Autodesk Inventor part; units mm, degrees
ref_plane "YZ Plane" through (0, 0, 0) normal (1, 0, 0) x (0, 1, 0)
ref_plane "XZ Plane" through (0, 0, 0) normal (0, 1, 0) x (-1, 0, 0)
ref_plane "XY Plane" through (0, 0, 0) normal (0, 0, 1) x (1, 0, 0)
sketch "Sketch1" plane through (0, 0, 0) normal (0, 0, 1) x (1, 0, 0)
  arc A0 (10, 32.7) -> (-10, 32.7) centre (0, 32.7) ccw
  line L0 (-10, 32.7) -> (-26, 14)
  line L1 (-26, 14) -> (-26, 7)
  line L2 (-26, 7) -> (-40, 7)
  line L3 (-40, 7) -> (-40, 0)
  line L4 (-40, 0) -> (0, 0)
  line L5 (0, 32.7) -> (0, 0) construction
  line L6 (10, 32.7) -> (26, 14)
  line L7 (26, 14) -> (26, 7)
  line L8 (26, 7) -> (40, 7)
  line L9 (40, 7) -> (40, 0)
  line L10 (40, 0) -> (0, 0)
  line L11 (-10, 32.7) -> (10, 32.7) construction
  dimension "d4" = 10
  dimension "d5" = 80
  dimension "ToolGuidance_Base_Thickness" = 7
  dimension "d7" = 7
  dimension "d8" = 32.7
  dimension "d9" = 14
  dimension "d11" = 0
extrude "Extrusion1" add sketch "Sketch1" against normal blind 60
sketch "Sketch2" plane through (0, 0, 0) normal (0, 0, 1) x (1, 0, 0)
  arc A0 (10, 32.7) -> (-10, 32.7) centre (0, 32.7) ccw
  circle A1 centre (0, 32.7) radius 8
  point P0 (0, 0)
  dimension "d16" = 16
extrude "Extrusion2" cut sketch "Sketch2" against normal blind 20
sketch "Sketch3" plane through (0, 0, -60) normal (0, 0, -1) x (-1, 0, 0)
  circle A0 centre (0, 32.7) radius 8
  circle A1 centre (0, 32.7) radius 4.25
  point P0 (0, 0)
  dimension "d19" = 8.5
extrude "Extrusion3" cut sketch "Sketch3" against normal blind 60 contours A1
sketch "Sketch4" plane through (-40, 7, 0) normal (0, 1, 0) x (1, 0, 0)
  circle A0 centre (5, 52) radius 2.25 construction
  line L0 (0, 60) -> (14, 60) construction
  line L1 (0, 0) -> (0, 60) construction
  circle A1 centre (5, 8) radius 2.25 construction
  line L2 (96, 0) -> (-16, 0) construction
  line L3 (40, 60) -> (40, 0) construction
  circle A2 centre (75, 52) radius 2.25 construction
  circle A3 centre (75, 8) radius 2.25 construction
  line L4 (80, 0) -> (80, 60) construction
  line L5 (66, 60) -> (80, 60) construction
  line L6 (75, 52) -> (75, 8) construction
  line L7 (5, 52) -> (5, 8) construction
  line L8 (0, 0) -> (0, 60) construction
  point P0 (73, 60)
  point P1 (7, 60)
  dimension "d25" = 4.5
  dimension "d26" = 8
  dimension "d28" = 4.5
  dimension "d29" = 8
  dimension "d54" = 44
  dimension "Guidacne_fixHoleDist" = 70
hole "Bohrung1" at (35, 7, -52) at (35, 7, -8) at (-35, 7, -8) at (-35, 7, -52) direction (0, -1, 0) diameter 3.4 end through all counterbore diameter 6.5 counterbore depth 3.4
sketch "Sketch5" plane through (0, 0, 0) normal (1, 0, 0) x (0, 1, 0)
  line L0 (32.7, 0) -> (32.7, -60)
  line L1 (32.7, 0) -> (32.7, -180.9299)
  line L2 (32.7, -60) -> (42.7, -60)
  line L3 (42.7, -60) -> (38.95, -110)
  line L4 (38.95, -110) -> (38.95, -155)
  line L5 (36.95, -60) -> (36.95, -20)
  line L6 (36.95, -60) -> (36.95, -155)
  line L7 (36.95, -155) -> (38.95, -155)
  line L8 (42.7, 0) -> (32.7, 0)
  point P0 (0, 0)
  dimension "d34" = 2
  dimension "d35" = 155
  dimension "d36" = 110
revolve "Revolution1" add sketch "Sketch5" angle 360 about axis through (0, 32.7, 0) along (0, 0, -1)
sketch "Sketch6" plane through (0, 0, 0) normal (1, 0, 0) x (0, 1, 0)
  line L0 (32.7, 0) -> (32.7, -60)
  line L1 (32.7, -41.8536) -> (32.7, 16.9969)
  line L2 (24.7, -20) -> (40.7, -20)
  line L3 (40.7, -20) -> (36.95, -33.9952)
  line L4 (36.95, -155) -> (36.95, -20)
  line L5 (28.45, -20) -> (36.95, -20)
  line L6 (36.95, -33.9952) -> (36.95, -20)
  line L7 (36.95, -20) -> (40.7, -20)
  line L8 (36.95, -33.9952) -> (36.95, -20)
  line L9 (40.7, -20) -> (36.95, -20)
  point P0 (0, 0)
  dimension "d38" = 15
revolve "Revolution2" cut sketch "Sketch6" angle 360 about axis through (0, 32.7, -41.8536) along (0, 0, 1)
sketch "Sketch7" plane through (0, 0, 0) normal (1, 0, 0) x (0, 1, 0)
  line L0 (26.45, -110) -> (38.95, -110)
  line L1 (32.7, -110) -> (32.7, -160.0229)
  line L2 (38.95, -110) -> (38.95, -155)
  line L3 (38.95, -122) -> (38.85, -122)
  line L4 (38.85, -122) -> (38.85, -130)
  line L5 (38.85, -130) -> (38.95, -130)
  line L6 (38.95, -130) -> (38.95, -122)
  line L7 (42.7, 0) -> (32.7, 0)
  point P0 (0, 0)
  dimension "d40" = 0.1
  dimension "d41" = 122
  dimension "d42" = 8
revolve "Revolution3" cut sketch "Sketch7" angle 360 about axis through (0, 32.7, -110) along (0, 0, -1)
ref_plane "Arbeitsebene1" through (0, 32.7, -126) normal (0, 0, -1) x (-1, 0, 0)
ref_plane "Arbeitsebene2" through (26, 7, 0) normal (0, 0, 1) x (1, 0, 0)
chamfer "Fase2" distance 6 angle 45 2 edges at (-40, 3.5, -60) (40, 3.5, -60)
sketch "Skizze9" plane through (-40, 0, 0) normal (0, -1, 0) x (1, 0, 0)
  circle A0 centre (5, -52) radius 1.7
  circle A1 centre (75, -8) radius 1.7
  circle A2 centre (75, -52) radius 1.7
  circle A3 centre (5, -8) radius 1.7
  line L0 (80, -54) -> (74, -60)
  line L1 (80, 0) -> (80, -54)
  line L2 (0, 0) -> (80, 0)
  line L3 (0, 0) -> (0, -54)
  line L4 (6, -60) -> (0, -54)
  line L5 (74, -60) -> (6, -60)
  point P0 (40, 0)
equation "\"d5\" = GuidanceTrac_Width"
equation "\"d25\" = d28"
properties part number "Guide" material "PBT-Kunststoff"
The model under review builds one solid part; all positions refer to its coordinate system, in mm. A direction names the side the tool comes from. Round coordinates to 2 decimals unless told otherwise and drop trailing zeros. Loops run counter-clockwise (first coordinate to the right, second up) from the corner with the lowest first, then second, coordinate; pieces in that order, holes last.
Item 1: For line 1 (X direction, y = 2.8, z = -8); line 2 (X direction, y = 4.4, z = -8); line 3 (Z direction, x = 35, y = 2.5), list the stretches that pass through material, from the lowest coordinate up.
Determined:
line 1: x = -40 to -36.7, -33.3 to 33.3, 36.7 to 40
line 2: x = -40 to -38.25, -31.75 to 31.75, 38.25 to 40
line 3: z = -59 to -53.7, -50.3 to -9.7, -6.3 to 0
Item 2: Clearance check with flat-ended pins moving along their axes: pin 1 Ø8 at (y, z) = (30, -29.5) entering from +X; pin 2 Ø4 at (x, y) = (-23.5, 18) entering from -Z; pin 3 Ø4 at (x, z) = (-32.5, -28.5) entering from +Y; pin 4 Ø10 at (x, y) = (7, 34) entering from -Z. State where each tip first meets the part, or that it passes through.
Determined:
pin 1: stops at x = 15.73
pin 2: stops at z = -60
pin 3: stops at y = 7
pin 4: stops at z = -155
Item 3: Take a section at C-C (x = -30). Write out the cut boundary in (y, z).
Determined:
outline: (0, -60) - (7, -60) - (7, 0) - (0, 0) - close
Item 4: Mouldability with a two-part tool opening along Y and no side actions: class faces 6 (the face through (-3.34, 30.07, -95.34)), 7 (the face through (37, 3, -57)), 8 (the face through (-2.36, 38.38, -126.06)) as released by +Y, released by -Y, zero draft, split by the parting line, or undercut.
Determined:
face 6: undercut
face 7: zero draft
face 8: split by the parting line
Item 5: Take a section at B-B (z = -40.5). Write out the cut boundary in (x, y), then the cut area to 3 significant figures.
Determined:
outline: (-40, 0) - (40, 0) - (40, 7) - (26, 7) - (26, 14) - (10, 32.7) arc R10 ccw to (-10, 32.7) - (-26, 14) - (-26, 7) - (-40, 7) - close; hole circle Ø8.5 at (0, 32.7)
area: 1,700 mm2
Item 6: Take a section at A-A (z = -8). Write out the cut boundary in (x, y).
Determined:
outline: (-40, 0) - (-36.7, 0) - (-36.7, 3.6) - (-38.25, 3.6) - (-38.25, 7) - (-40, 7) - close; (-33.3, 0) - (33.3, 0) - (33.3, 3.6) - (31.75, 3.6) - (31.75, 7) - (26, 7) - (26, 14) - (10, 32.7) arc R10 ccw to (-10, 32.7) - (-26, 14) - (-26, 7) - (-31.75, 7) - (-31.75, 3.6) - (-33.3, 3.6) - close; (36.7, 0) - (40, 0) - (40, 7) - (38.25, 7) - (38.25, 3.6) - (36.7, 3.6) - close; hole circle Ø16 at (0, 32.7)
Item 7: Take a section at D-D (z = -141). Write out the cut boundary in (x, y).
Determined:
outline: circle Ø12.5 at (0, 32.7); hole circle Ø8.5 at (0, 32.7)
Item 8: For faces 1 (the face through (0.275, 26.456, -142.675)), 2 (the face through (-26, 11, -30)), 3 (the face through (-1, 37, -155)), 4 (the face through (36.4, 3.6, -50.6)), 5 (the face through (-1.73, 24.89, -9.86)), list the 3-axis set-ups (+Z, -Z, +X, -X, +Y, -Y) from which the entire face can be reached by the end or side of a thin tool; tool diameter is ignored.
Determined:
face 1: -Z
face 2: +Z, -Z, -X, +Y
face 3: -Z, +X, -X, +Y, -Y
face 4: +Y
face 5: +Z
